from build123d import *

# Parameters (mm, degrees)
BOSS_EXTRU_1_DEPTH                        = 40
ESQUISSE2_W                               = 1
ESQUISSE2_H                               = 30
EXTRU_MINCE2_DEPTH                        = 1
R_P_TITION_LIN_AIRE1_COUNT                = 12
R_P_TITION_LIN_AIRE1_PITCH                = 3
TROU_POUR_TARAUDAGE_POUR_TROU_TARAUD_M3_D = 2.5
D_GAGEMENT_M33_D                          = 3.6


with BuildPart() as part:
    # Esquisse1 → Boss.-Extru.1 (new body)
    with BuildSketch(Plane.XY):
        Polygon((-17.178456592, 11.666666667), (-17.178456592, -18.333333333), (17.821543408, -18.333333333), (17.821543408, -13.333333333), (-12.178456592, -13.333333333), (-12.178456592, 11.666666667), align=None)
    extrude(amount=BOSS_EXTRU_1_DEPTH)

    # Esquisse2 → Extru.-Mince2 (add)
    with BuildSketch(Plane.ZY.offset(17.178456592)):
        with Locations((36.5, -3.333333333)):
            Rectangle(ESQUISSE2_W, ESQUISSE2_H)
    extru_mince2 = extrude(amount=EXTRU_MINCE2_DEPTH)

    # Répétition linéaire1: Extru.-Mince2 ×12
    with Locations(*[(0, 0, -i * R_P_TITION_LIN_AIRE1_PITCH) for i in range(1, R_P_TITION_LIN_AIRE1_COUNT)]):
        add(extru_mince2)

    # Trou pour taraudage pour trou taraudé M34 (through all)
    with Locations(Plane(origin=(-12.178456592, 0, 0), x_dir=(0, 0, -1), z_dir=(1, 0, 0))):
        with Locations((-5, 6.666666667), (-35, 6.666666667), (-35, -8.333333333), (-5, -8.333333333)):
            Hole(TROU_POUR_TARAUDAGE_POUR_TROU_TARAUD_M3_D / 2)

    # Dégagement M33 (through all)
    with Locations(Plane(origin=(0, -13.333333333, 0), x_dir=(1, 0, 0), z_dir=(0, 1, 0))):
        with Locations((14.821543408, -10), (14.821543408, -30), (-5.178456592, -10), (-5.178456592, -30)):
            Hole(D_GAGEMENT_M33_D / 2)


solid = part.part
Build history of the part. All positions in model axes, mm. A direction names the side the tool comes from. Give positions to 0.01 mm unless a question says otherwise; leave off trailing zeros. Write each loop counter-clockwise with the first axis right and the second up, starting at its lowest first coordinate (ties: lowest second). Pieces come first, ordered by that corner, then holes. Notation, with made-up numbers: (67.25, -25) - (81.25, -25) arc R38 cw to (81.25, 13) - close; hole circle Ø9 at (89.25, -37.75). An arc over 180 degrees is marked (long way). Use one line per item in the form item = value. Start each with the question number.
1. Band-saw the part on C-C on x = 14. Write the cut outline in (y, z), plus the area to 3 significant figures.
2. 3-axis set-ups, long thin cutter, end or side, ignore diameter. For faces 4 (the face through (-18, -4, 22)), 5 (the face through (-18, -4, 3)), 6 (the face through (-12.178, -1, 20)), 7 (the face through (-14.554, 7.042, 36.192)): which of +Z, -Z, +X, -X, +Y, -Y reach the whole face in a straight line?
3. Band-saw the part on D-D on z = 19.5. Write the cut outline in (x, y), plus the area to 3 significant figures.
4. Band-saw the part on B-B on x = -14. Write the cut outline in (y, z).
5. Two-plate mould, pull along Z, no slides. Class faces 1 (the face through (-14.554, -7.958, 6.192)), 2 (the face through (-6, -14, 0)), 3 (the face through (-18.178, -3.1, 15.5)): released by +Z, released by -Z, zero draft, split by the parting line, or undercut.
6. Band-saw the part on A-A on z = 5. Write the cut outline in (x, y), plus the area to 3 significant figures.
7. Drop flat-ended pins along their axis: pin 1 Ø1.5 at (x, z) = (0.5, 7) entering from +Y; pin 2 Ø5 at (y, z) = (4, 12.5) entering from +X; pin 3 Ø1.1 at (x, y) = (-18, -2.5) entering from +Z. Give the stop position or say it passes through.
8. Probe line 1 (Y direction, x = -13, z = 5); line 2 (Z direction, x = -16, y = 6); line 3 (X direction, y = -14, z = 32). List the from-to ranges inside material, lowest first. Write a range as [from, to].
Conclusion:
q1.outline = (-18.33, 0) - (-13.33, 0) - (-13.33, 8.4) - (-18.33, 8.4) - close; (-18.33, 11.6) - (-13.33, 11.6) - (-13.33, 28.4) - (-18.33, 28.4) - close; (-18.33, 31.6) - (-13.33, 31.6) - (-13.33, 40) - (-18.33, 40) - close
q1.area = 168 mm²
q2.face_4 = -X, +Y, -Y
q2.face_5 = -Z, -X, +Y, -Y
q2.face_6 = +Z, -Z, +X, +Y
q2.face_7 = +X, -X
q3.outline = (-17.18, -18.33) - (17.82, -18.33) - (17.82, -13.33) - (-12.18, -13.33) - (-12.18, 11.67) - (-17.18, 11.67) - close
q3.area = 300 mm²
q4.outline = (-18.33, 0) - (11.67, 0) - (11.67, 40) - (-18.33, 40) - close; hole circle Ø2.5 at (-8.33, 5); hole circle Ø2.5 at (-8.33, 35); hole circle Ø2.5 at (6.67, 5); hole circle Ø2.5 at (6.67, 35)
q5.face_1 = undercut
q5.face_2 = released by -Z
q5.face_3 = zero draft
q6.outline = (-17.18, -18.33) - (17.82, -18.33) - (17.82, -13.33) - (-12.18, -13.33) - (-12.18, -9.58) - (-17.18, -9.58) - close; (-17.18, -7.08) - (-12.18, -7.08) - (-12.18, 5.42) - (-17.18, 5.42) - close; (-17.18, 7.92) - (-12.18, 7.92) - (-12.18, 11.67) - (-17.18, 11.67) - close
q6.area = 275 mm²
q7.pin_1 = -13.33
q7.pin_2 = -12.18
q7.pin_3 = 37
q8.line_1 = [-18.33, -9.58], [-7.08, 5.42], [7.92, 11.67]
q8.line_2 = [0, 3.94], [6.06, 33.94], [36.06, 40]
q8.line_3 = [-17.18, 17.82]
